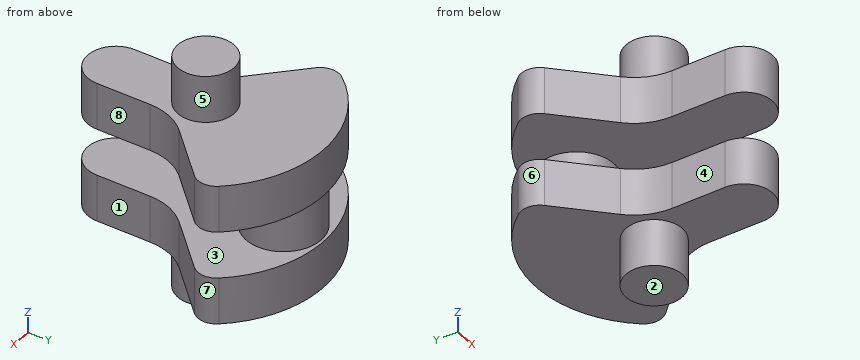
from build123d import *

# Parameters (mm, degrees)
BOSS_EXTRUDE1_DEPTH = 37.5
FILLET1_R           = 10
SKETCH4_W           = 25
SKETCH4_H           = 105.707635496
FILLET2_R           = 30
SKETCH5_R           = 15
BOSS_EXTRUDE2_DEPTH = 25


with BuildPart() as part:
    # Sketch2 → Boss-Extrude1 (new body, symmetric)
    with BuildSketch(Plane.XY):
        with BuildLine():
            Line((15, -47.5), (15, -7))
            Line((15, -7), (53.80332931, 31.80332931))
            ThreePointArc((53.80332931, 31.80332931), (0, 62.5), (-53.80332931, 31.80332931))
            Line((-53.80332931, 31.80332931), (-15, -7))
            Line((-15, -7), (-15, -47.5))
            ThreePointArc((-15, -47.5), (0, -62.5), (15, -47.5))
        make_face()
    extrude(amount=BOSS_EXTRUDE1_DEPTH, both=True)

    # Fillet1
    fillet1_edges = [part.edges().sort_by_distance(p)[0] for p in [
        (-53.80332931, 31.80332931, 0),
        (53.80332931, 31.80332931, 0),
    ]]
    fillet(fillet1_edges, radius=FILLET1_R)

    # Sketch4 → Cut-Revolve1 (revolve, cut)
    with BuildSketch(Plane(origin=(0, 0, 0), x_dir=(0, 0, -1), z_dir=(1, 0, 0)), mode=Mode.PRIVATE) as cut_revolve1_sk:
        with Locations((0, -31.853817748)):
            Rectangle(SKETCH4_W, SKETCH4_H)
    revolve(cut_revolve1_sk.sketch.rotate(Axis((0, 41, 37.5), (0, 0, -1)), 270), axis=Axis((0, 41, 37.5), (0, 0, -1)), mode=Mode.SUBTRACT)  # turned: the seam where the file's is

    # Fillet2
    fillet2_edges = [part.edges().sort_by_distance(p)[0] for p in [
        (15, -7, 25),
        (-15, -7, 25),
        (15, -7, -25),
        (-15, -7, -25),
    ]]
    fillet(fillet2_edges, radius=FILLET2_R)

    # Sketch5 → Boss-Extrude2 (add)
    with BuildSketch(Plane.XY.offset(37.5)):
        Circle(SKETCH5_R)
    boss_extrude2 = extrude(amount=BOSS_EXTRUDE2_DEPTH)

    # Mirror1: Boss-Extrude2 across plane
    add(boss_extrude2.mirror(Plane.XY))


solid = part.part
The model under review builds one solid part; all positions refer to its coordinate system, in mm. Face numbers are marked on the shaded views. A direction names the side the tool comes from. Round coordinates to 2 decimals unless told otherwise and drop trailing zeros. Write each loop counter-clockwise with the first axis right and the second up, starting at its lowest first coordinate (ties: lowest second). Pieces come first, ordered by that corner, then holes. Notation, with made-up numbers: (-25, 88.5) -> (-11, 88.5) arc R31 ccw to (-11, 126.5) -> close; hole circle Ø4 at (38.5, -21.5). An arc over 180 degrees is marked (long way). Answer as a JSON object with one key per item and string values.
1. Machinability: for the marked faces 4, 5, 6, 7 and 8, which of the approach directions +Z, -Z, +X, -X, +Y, -Y give a long, thin tool a straight path to every point of the face, cutting with its end or side? Answer none if there is none.
Results found:
{"face 4": "+Z, -Z, -X, -Y", "face 5": "+Z", "face 6": "+Z, -Z, -X", "face 7": "+Z, -Z, +X", "face 8": "+Z, -Z, +X, -Y"}
2. We need section A-A on y = -39. State the section outline as (x, z) points.
Results found:
{"outline": "(-15, -37.5) -> (15, -37.5) -> (15, -12.5) -> (-15, -12.5) -> close; (-15, 12.5) -> (15, 12.5) -> (15, 37.5) -> (-15, 37.5) -> close"}
3. The part is to be moulded in two halves that separate along Z. For the marked faces 1, 2 and 3, say which applies: pulls with the +Z half, pulls with the -Z half, needs draft (parallel to the pull), parting line crosses it, or undercut.
Results found:
{"face 1": "needs draft", "face 2": "pulls with the -Z half", "face 3": "undercut"}
4. We need section B-B on z = -21. State the section outline as (x, y) points.
Results found:
{"outline": "(-48.62, 39.27) arc R10 ccw to (-47.91, 25.91) -> (-23.79, 1.79) arc R30 cw to (-15, -19.43) -> (-15, -47.5) arc R15 ccw to (15, -47.5) -> (15, -19.43) arc R30 cw to (23.79, 1.79) -> (47.91, 25.91) arc R10 ccw to (48.62, 39.27) arc R62.5 ccw to start"}
5. We need section D-D on x = 0. State the section outline as (y, z) points.
Results found:
{"outline": "(-62.5, -37.5) -> (-15, -37.5) -> (-15, -62.5) -> (15, -62.5) -> (15, -37.5) -> (62.5, -37.5) -> (62.5, -12.5) -> (61, -12.5) -> (61, 12.5) -> (62.5, 12.5) -> (62.5, 37.5) -> (15, 37.5) -> (15, 62.5) -> (-15, 62.5) -> (-15, 37.5) -> (-62.5, 37.5) -> (-62.5, 12.5) -> (21, 12.5) -> (21, -12.5) -> (-62.5, -12.5) -> close"}
6. We need section C-C on x = -28. State the section outline as (y, z) points.
Results found:
{"outline": "(6, -37.5) -> (55.88, -37.5) -> (55.88, -12.5) -> (6, -12.5) -> close; (6, 12.5) -> (55.88, 12.5) -> (55.88, 37.5) -> (6, 37.5) -> close"}
7. Clearance check with flat-ended pins moving along their axes: pin 1 (4 mm diameter, centred on x = -14.5, y = 15.5, fed in from -Z); pin 2 (10 mm diameter, centred on y = 3.5, z = 11.5, fed in from -X); pin 3 (10 mm diameter, centred on x = 23, z = 41, fed in from -Y). State where each tip first meets the part, or that it passes through.
Results found:
{"pin 1": "stops at z = -37.5", "pin 2": "stops at x = -30.4", "pin 3": "stops at y = -3.74"}
8. To check wall thickness, follow line 1 along Z through (x, y) = (26, 40.5); line 2 along Z through (x, y) = (-1.5, 13.5); line 3 along X through (y, z) = (-42.5, -29). State the ranges of each line that lie inside material, in increasing order.
Results found:
{"line 1": "z = -37.5 to -12.5, 12.5 to 37.5", "line 2": "z = -62.5 to -12.5, 12.5 to 62.5", "line 3": "x = -15 to 15"}
